from build123d import *

# Parameters (mm, degrees)
SKETCH1_W           = 12.7
SKETCH1_H           = 9.525
BOSS_EXTRUDE1_DEPTH = 2.54
FILLET1_R           = 0.635
SHELL1_START        = 0.635
SHELL1_OUTLINE_W    = 1.905
SHELL1_OUTLINE_H    = 8.255
SHELL1_DEPTH        = 11.43
SKETCH2_R           = 2.54
BOSS_EXTRUDE2_DEPTH = 1.905
BOSS_EXTRUDE3_DEPTH = 0.00254


# Read off the part's stored shape, not the designer's step: Shell1
with BuildPart() as part:
    # Sketch1 → Boss-Extrude1 (new body)
    with BuildSketch(Plane(origin=(0, 0, 0), x_dir=(1, 0, 0), z_dir=(0, 1, 0))):
        with Locations((6.35, 4.7625)):
            Rectangle(SKETCH1_W, SKETCH1_H)
    extrude(amount=BOSS_EXTRUDE1_DEPTH)

    # Fillet1
    fillet1_edges = [part.edges().sort_by_distance(p)[0] for p in [
        (0, 1.27, -9.525),
        (12.7, 1.27, -9.525),
        (12.7, 1.27, 0),
        (0, 1.27, 0),
    ]]
    fillet(fillet1_edges, radius=FILLET1_R)

    # Shell1 outline → Shell1 (cut)
    with BuildSketch(Plane.YZ.offset(SHELL1_START)):
        with Locations((0.9525, -4.7625)):
            Rectangle(SHELL1_OUTLINE_W, SHELL1_OUTLINE_H)
    extrude(amount=SHELL1_DEPTH, mode=Mode.SUBTRACT)

    # Sketch2 → Boss-Extrude2 (add)
    with BuildSketch(Plane(origin=(0, 1.905, 0), x_dir=(-1, 0, 0), z_dir=(0, -1, 0))):
        with Locations(Location((-6.35, 4.7625, 0), (0, 0, 270))):
            Circle(SKETCH2_R)
    extrude(amount=BOSS_EXTRUDE2_DEPTH)

    # Sketch3 → Boss-Extrude3 (add)
    with BuildSketch(Plane(origin=(0, 2.54, 0), x_dir=(1, 0, 0), z_dir=(0, 1, 0))):
        Polygon((4.557346154, 6.477), (6.104141026, 6.477), (6.104141026, 5.907128205), (5.127217949, 5.907128205), (5.127217949, 5.296551282), (6.104141026, 5.296551282), (6.104141026, 4.726679487), (5.127217949, 4.726679487), (5.127217949, 3.302), (4.557346154, 3.302), align=None)
        with BuildLine():
            Line((7.040358974, 5.418666667), (6.470487179, 5.418666667))
            add(Edge.make_bspline(
                [(6.470487179, 5.418666667), (6.472948368, 5.461774453), (6.477757384, 5.54600448), (6.496886431, 5.66835129), (6.522518698, 5.783955572), (6.556728361, 5.89241293), (6.599715041, 5.993683952), (6.65037258, 6.088113879), (6.709995163, 6.175205533), (6.777313826, 6.254538911), (6.851185682, 6.325709616), (6.930077079, 6.388814034), (7.015194768, 6.440886212), (7.104983579, 6.483736794), (7.199428222, 6.517972417), (7.299422293, 6.540861702), (7.404099988, 6.55636255), (7.475760347, 6.557718936), (7.512284054, 6.558410256)],
                knots=[0, 0, 0, 0, 1.199038563, 2.342849363, 3.436047546, 4.486744587, 5.497670872, 6.488682221, 7.459191391, 8.424610317, 9.374430501, 10.305433194, 11.225809216, 12.140057399, 13.06607119, 14.010487599, 14.985989317, 16, 16, 16, 16], degree=3))
            add(Edge.make_bspline(
                [(7.512284054, 6.558410256), (7.557116388, 6.557011369), (7.644639608, 6.554280414), (7.77181779, 6.53098446), (7.890588306, 6.492018376), (8.000864822, 6.437572481), (8.101708535, 6.368404679), (8.193102721, 6.285933395), (8.272283476, 6.188428338), (8.339752827, 6.079946535), (8.395811794, 5.965079574), (8.435095583, 5.846302372), (8.460916395, 5.726766795), (8.463670345, 5.646277588), (8.465038462, 5.606291867)],
                knots=[0, 0, 0, 0, 1.075374347, 2.099382735, 3.09057751, 4.06680945, 5.040638231, 6.016817125, 7.011024321, 8.044445721, 9.0776792, 10.070479129, 11.0414456, 12, 12, 12, 12], degree=3))
            add(Edge.make_bspline(
                [(8.465038462, 5.606291867), (8.464505789, 5.582105677), (8.463433651, 5.53342485), (8.455978932, 5.459758812), (8.44479538, 5.384721339), (8.427933309, 5.308376769), (8.406904924, 5.230703702), (8.381394454, 5.151469689), (8.350810158, 5.071123958), (8.315662426, 4.98876223), (8.273731092, 4.904117111), (8.224907883, 4.815919737), (8.167896919, 4.724248345), (8.103386822, 4.62858533), (8.03106428, 4.529081566), (7.950576239, 4.426036789), (7.862849733, 4.319087904), (7.800587764, 4.247598577), (7.768599159, 4.210869191)],
                knots=[0, 0, 0, 0, 0.728284026, 1.46585585, 2.227944881, 3.01186502, 3.81876927, 4.650621989, 5.517437689, 6.406905708, 7.346299482, 8.360816762, 9.441613733, 10.596154504, 11.834900912, 13.145207542, 14.533280747, 16, 16, 16, 16], degree=3))
            Line((7.768599159, 4.210869191), (7.437233974, 3.831166667))
            Line((7.437233974, 3.831166667), (8.50574359, 3.831166667))
            Line((8.50574359, 3.831166667), (8.50574359, 3.302))
            Line((8.50574359, 3.302), (6.389076923, 3.302))
            Line((6.389076923, 3.302), (6.389076923, 3.590752003))
            Line((6.389076923, 3.590752003), (7.329110978, 4.591207732))
            add(Edge.make_bspline(
                [(7.329110978, 4.591207732), (7.356327379, 4.620391337), (7.409037478, 4.676911324), (7.484038516, 4.759916937), (7.551907831, 4.838687284), (7.611238096, 4.914061108), (7.665142888, 4.983593589), (7.711218596, 5.049380524), (7.749886777, 5.110827174), (7.791866571, 5.184921103), (7.831733577, 5.273291298), (7.868313967, 5.375097387), (7.890612246, 5.47240056), (7.893690114, 5.5358054), (7.895166667, 5.566222756)],
                knots=[0, 0, 0, 0, 1.246127091, 2.413378631, 3.493388633, 4.492180848, 5.408488754, 6.240484944, 6.999099869, 7.674939598, 8.898438119, 10.020720584, 11.050475521, 12, 12, 12, 12], degree=3))
            add(Edge.make_bspline(
                [(7.895166667, 5.566222756), (7.894062684, 5.595649202), (7.89192354, 5.652667658), (7.868416082, 5.733776109), (7.831997512, 5.807211531), (7.780678605, 5.870779591), (7.718515335, 5.923017682), (7.646679837, 5.961870906), (7.565757782, 5.984289038), (7.50902988, 5.987094988), (7.479847155, 5.988538462)],
                knots=[0, 0, 0, 0, 1.062038974, 2.057870785, 3.028805853, 4.01125022, 4.991535629, 5.949134679, 6.94496649, 8, 8, 8, 8], degree=3))
            add(Edge.make_bspline(
                [(7.479847155, 5.988538462), (7.464770988, 5.988005225), (7.435091132, 5.986955463), (7.391464063, 5.979967483), (7.349949772, 5.967651898), (7.310086183, 5.951150747), (7.27229873, 5.929278353), (7.236682725, 5.902317143), (7.202862908, 5.870952262), (7.170994391, 5.835281784), (7.14198988, 5.79547352), (7.116228179, 5.751891037), (7.094927542, 5.704561389), (7.076173686, 5.654109398), (7.061709815, 5.59999317), (7.051178323, 5.542536583), (7.043171933, 5.481833113), (7.041313685, 5.440105185), (7.040358974, 5.418666667)],
                knots=[0, 0, 0, 0, 0.903469896, 1.778625579, 2.63899355, 3.493148037, 4.358286772, 5.247621495, 6.164656832, 7.118446693, 8.109501108, 9.111810964, 10.146451449, 11.215617525, 12.33435995, 13.498009769, 14.714554818, 16, 16, 16, 16], degree=3))
        make_face()
    extrude(amount=BOSS_EXTRUDE3_DEPTH)


solid = part.part
Source: CAD feature listing. Evaluate the final solid. Frame: model axes, mm. A direction names the side the tool comes from. Give positions to 0.01 mm unless a question says otherwise; leave off trailing zeros. Write each loop counter-clockwise with the first axis right and the second up, starting at its lowest first coordinate (ties: lowest second). Pieces come first, ordered by that corner, then holes. Notation, with made-up numbers: M 86,5.5 L 98,5.5 A29 ccw 98,26.5 Z; hole C -12,52.25 d8. An arc over 180 degrees is marked long. Answer as a JSON object with one key per item and string values.
Q1. Cut plane B-B, the plane x = 2. Return the cut outline in (y, z) (3 decimals).
Geometry check:
{"outline": "M 0,-9.525 L 2.54,-9.525 L 2.54,0 L 0,0 L 0,-0.635 L 1.905,-0.635 L 1.905,-8.89 L 0,-8.89 Z"}
Q2. Cut plane D-D, the plane z = -7. Return the cut outline in (x, y) (3 decimals).
Geometry check:
{"outline": "M 0,0 L 0.635,0 L 0.635,1.905 L 5.148,1.905 L 5.148,0 L 7.552,0 L 7.552,1.905 L 12.065,1.905 L 12.065,0 L 12.7,0 L 12.7,2.54 L 0,2.54 Z"}
Q3. Cut plane A-A, the plane y = 1.4. Count the separate pieces of the cut face and the enclosed holes in it, then the cut area to 3 significant figures.
Geometry check:
{"separate pieces": "2", "enclosed holes": "1", "area": "46.5 mm^2"}
Q4. Access query for faces 1 (the face through (8, 2.543, -5)), 2 (the face through (6, 1, -0.635)). Directions: +Z, -Z, +X, -X, +Y, -Y. A direction counts if a zero-diameter tool reaches every point of the face in a straight line with its end or side. Return the directions, or none.
Geometry check:
{"face 1": "+Z, -Z, +X, -X, +Y", "face 2": "-Y"}
Q5. Mould query, pull axis Z, two halves, no side actions, for faces 3 (the face through (0, 1, -5)), 4 (the face through (12.065, 1, -5)), 5 (the face through (6, 1, -9.525)). Classes: +Z half, -Z half, draft (parallel to the pull), parting line (faces both ways), or undercut.
Geometry check:
{"face 3": "draft", "face 4": "undercut", "face 5": "-Z half"}
Q6. Ray query, line 1 along Z through (x, y) = (3.5, 0.55) (3 decimals); line 2 along X through (y, z) = (1.65, -4.25) (3 decimals); line 3 along X through (y, z) = (1.7, -8.5) (3 decimals). Return the intervals inside material, ascending.
Geometry check:
{"line 1": "z = -9.525 to -8.89, -0.635 to 0", "line 2": "x = 0 to 0.635, 3.862 to 8.838, 12.065 to 12.7", "line 3": "x = 0 to 0.635, 12.065 to 12.7"}
Q7. Cut plane C-C, the plane z = -1.25. Return the cut outline in (x, y) (3 decimals), then the cut area to 3 significant figures.
Geometry check:
{"outline": "M 0,0 L 0.635,0 L 0.635,1.905 L 12.065,1.905 L 12.065,0 L 12.7,0 L 12.7,2.54 L 0,2.54 Z", "area": "10.5 mm^2"}
